The figure shows three views and two pictorial views of one solid part (mm, origin at its lowest corner). Answer the questions. Give positions to 0.01 mm unless a question says otherwise; leave off trailing zeros. Order: outer loops, then holes, each group sorted by start corner. A loop starts at its lowest first (then second) coordinate and runs counter-clockwise, first axis right, second up. Notation, with made-up numbers: M -38.75,-30.5 L -15.75,-30.5 A21 ccw -15.75,-24.5 Z; hole C -3.5,-13 d5. An arc over 180 degrees is marked long. One line per item, written item: value.
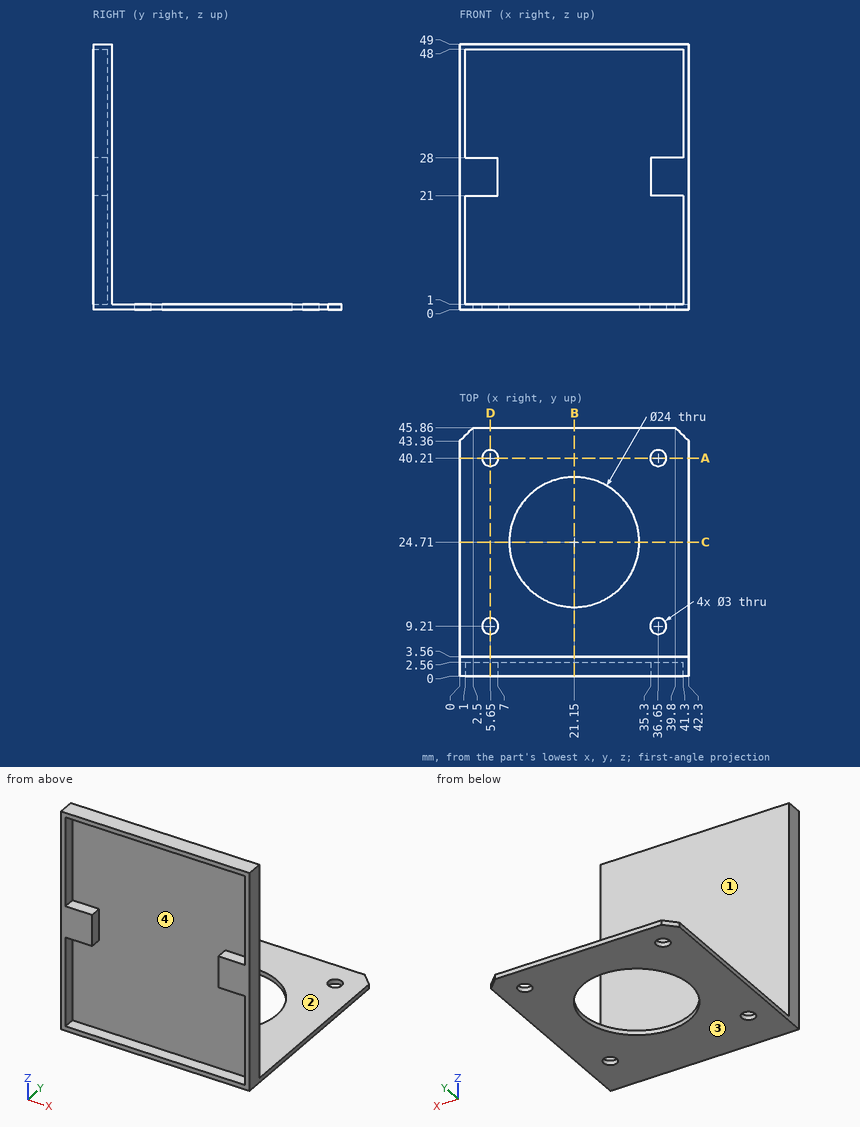
1) Find section B-B, the plane x = 21.15. Write down the section's boundary in (y, z), plus the area to 3 significant figures.
Reported:
outline: M 0,0 L 12.71,0 L 12.71,1 L 3.56,1 L 3.56,49 L 0,49 L 0,48 L 2.56,48 L 2.56,1 L 0,1 Z; M 36.71,0 L 45.86,0 L 45.86,1 L 36.71,1 Z
area: 72.4 mm^2
2) Each of these flat-tipped pins is pushed along its axis until it touches: pin 1 Ø5 at (x, z) = (7.5, 33.5) entering from +Y; pin 2 Ø3 at (x, y) = (4.5, 1.5) entering from -Z; pin 3 Ø19 at (x, y) = (21.15, 24.71) entering from +Z; pin 4 Ø10 at (x, z) = (26, 17) entering from -Y. Where does it stop, or does it pass through?
Reported:
pin 1: stops at y = 3.56
pin 2: stops at z = 0
pin 3: passes through
pin 4: stops at y = 2.56
3) Find section D-D, the plane x = 5.65. Write down the section's boundary in (y, z), plus the area to 3 significant figures.
Reported:
outline: M 0,0 L 7.71,0 L 7.71,1 L 3.56,1 L 3.56,49 L 0,49 L 0,48 L 2.56,48 L 2.56,28 L 0,28 L 0,21 L 2.56,21 L 2.56,1 L 0,1 Z; M 10.71,0 L 38.71,0 L 38.71,1 L 10.71,1 Z; M 41.71,0 L 45.86,0 L 45.86,1 L 41.71,1 Z
area: 108 mm^2
4) Consider probe 1 along Y at (x, z) = (5.65, 0.6); probe 2 along X at (y, z) = (2, 9); probe 3 along Y at (x, z) = (4.5, 4.5). Determine where each line is inside the solid, lowest interval first.
Reported:
probe 1: y = 0 to 7.71, 10.71 to 38.71, 41.71 to 45.86
probe 2: x = 0 to 1, 41.3 to 42.3
probe 3: y = 2.56 to 3.56
5) Find section C-C, the plane y = 24.71. Write down the section's boundary in (x, z), plus the area to 3 significant figures.
Reported:
outline: M 0,0 L 9.15,0 L 9.15,1 L 0,1 Z; M 33.15,0 L 42.3,0 L 42.3,1 L 33.15,1 Z
area: 18.3 mm^2
6) Find section A-A, the plane y = 40.21. Write down the section's boundary in (x, z).
Reported:
outline: M 0,0 L 4.15,0 L 4.15,1 L 0,1 Z; M 7.15,0 L 35.15,0 L 35.15,1 L 7.15,1 Z; M 38.15,0 L 42.3,0 L 42.3,1 L 38.15,1 Z
7) Determine the mould class of the marked faces 1, 2, 3 and 4 for opening direction Z: +Z half, -Z half, draft (parallel to the pull), parting line (faces both ways), or undercut.
Reported:
face 1: draft
face 2: +Z half
face 3: -Z half
face 4: undercut
